```python
from build123d import *

# Parameters (mm, degrees)
SKETCH1_R             = 1.6499999999999988
SKETCH1_R_2           = 1.6499999999999992
BOSS_EXTRUDE1_DEPTH   = 24
BOSS_EXTRUDE1_2_DEPTH = 24
SKETCH5_R             = 3.0000000000000044
SKETCH5_R_2           = 2.9999999999999996
CUT_EXTRUDE1_DEPTH    = 3
SKETCH6_W             = 2.999999999999975
SKETCH6_H             = 17.999999999999996
BOSS_EXTRUDE2_DEPTH   = 5
FILLET1_R             = 3
BOSS_EXTRUDE3_DEPTH   = 7
CHAMFER1_SIZE         = 2
FILLET2_R             = 0.6
FILLET3_R             = 1.2
CHAMFER2_SIZE         = 0.2
FILLET4_R             = 0.8


with BuildPart() as part:
    # Sketch1 → Boss-Extrude1 (new body)
    with BuildSketch(Plane.XY):
        with BuildLine():
            Line((-24.12157620169872, 10.3), (-9.293008124391159, 10.3))
            ThreePointArc((-9.293008124391159, 10.3), (-9.052493629563461, 10.342616719274229), (-8.841264673899918, 10.465277777777773))
            ThreePointArc((-8.84126467389991, 10.465277777777777), (-2.7566148708280886, 13.419801580274177), (4.000000000000017, 13.103053079339933))
            Line((4.000000000000019, 13.103053079339944), (4.000000000000019, 18))
            ThreePointArc((4.0000000000000195, 18), (1.4019415263376545, 21.7462728086366), (-3.0172799783650257, 20.626027709708623))
            ThreePointArc((-3.017279978365025, 20.626027709708623), (-5.396557983146459, 18.850985983990057), (-8.297519940503818, 18.221576201698717))
            Line((-8.297519940503818, 18.22157620169872), (-22, 18.221576201698717))
            ThreePointArc((-22, 18.221576201698717), (-26.540740078127286, 16.340740078127293), (-28.42157620169869, 11.799999999999997))
            Line((-28.42157620169869, 11.799999999999997), (-28.421576201698695, 8.999999999999998))
            Line((-28.421576201698695, 8.999999999999998), (-25.42157620169872, 8.999999999999998))
            ThreePointArc((-25.42157620169872, 8.999999999999998), (-25.040815017241233, 9.919238815542512), (-24.12157620169872, 10.3))
        make_face()
        with Locations((-21.999999999999996, 14)):
            Circle(SKETCH1_R, mode=Mode.SUBTRACT)
        with Locations((-6.49e-15, 18)):
            Circle(SKETCH1_R_2, mode=Mode.SUBTRACT)
    extrude(amount=BOSS_EXTRUDE1_DEPTH)


with BuildPart() as body_2:
    # Sketch1 → Boss-Extrude1 2 (new body)
    with BuildSketch(Plane.XY):
        with BuildLine():
            ThreePointArc((-24.12157620169872, -10.299999999999999), (-25.040815017241233, -9.91923881554251), (-25.42157620169872, -8.999999999999998))
            Line((-25.42157620169872, -8.999999999999998), (-28.421576201698723, -8.999999999999998))
            Line((-28.421576201698723, -8.999999999999998), (-28.42157620169872, -11.799999999999997))
            ThreePointArc((-28.42157620169872, -11.799999999999997), (-26.540740078127314, -16.340740078127318), (-21.999999999999996, -18.22157620169873))
            Line((-21.999999999999996, -18.22157620169873), (-8.297519940503813, -18.221576201698728))
            ThreePointArc((-8.297519940503813, -18.221576201698728), (-5.3965579831464545, -18.850985983990064), (-3.0172799783650195, -20.62602770970863))
            ThreePointArc((-3.0172799783650204, -20.62602770970863), (1.4019415263376571, -21.74627280863661), (4.000000000000004, -18))
            Line((4.000000000000004, -18), (4.000000000000004, -13.103053079339944))
            ThreePointArc((4.000000000000004, -13.103053079339945), (-2.756614870828109, -13.41980158027418), (-8.841264673899921, -10.465277777777775))
            ThreePointArc((-8.841264673899923, -10.465277777777775), (-9.052493629563463, -10.342616719274227), (-9.293008124391159, -10.299999999999999))
            Line((-9.293008124391159, -10.299999999999999), (-24.12157620169872, -10.299999999999999))
        make_face()
        with Locations((-21.999999999999996, -14)):
            Circle(SKETCH1_R, mode=Mode.SUBTRACT)
        with Locations((4.53e-15, -18)):
            Circle(SKETCH1_R_2, mode=Mode.SUBTRACT)
    extrude(amount=BOSS_EXTRUDE1_2_DEPTH)


with BuildPart() as cut_extrude1_tool:
    # Sketch5 → Cut-Extrude1 (new body)
    with BuildSketch(Plane.XY.offset(24)):
        with Locations((-21.999999999999996, 14)):
            Circle(SKETCH5_R)
        with Locations((-6.49e-15, 18)):
            Circle(SKETCH5_R_2)
        with Locations((4.53e-15, -18)):
            Circle(SKETCH5_R_2)
        with Locations((-21.999999999999996, -14)):
            Circle(SKETCH5_R)
    extrude(amount=-CUT_EXTRUDE1_DEPTH)


with BuildPart() as part_1:
    add(part.part)

    # Cut-Extrude1: cut by cut_extrude1_tool
    add(cut_extrude1_tool.part, mode=Mode.SUBTRACT)



with BuildPart() as body_2_1:
    add(body_2.part)

    # Cut-Extrude1: cut by cut_extrude1_tool
    add(cut_extrude1_tool.part, mode=Mode.SUBTRACT)


with BuildPart() as part_2:
    add(part_1.part)

    add(body_2_1.part)  # Boss-Extrude2 merges body 2
    # Sketch6 → Boss-Extrude2 (add)
    with BuildSketch(Plane.XY.offset(24)):
        with Locations((-26.921576201698706, 0)):
            Rectangle(SKETCH6_W, SKETCH6_H)
    extrude(amount=-BOSS_EXTRUDE2_DEPTH)

    # Fillet1
    fillet1_edges = [part_2.edges().sort_by_distance(p)[0] for p in [
        (4.000000000000018, 13.103053079339938, 12),
        (4.0000000000000036, -13.103053079339944, 12),
    ]]
    fillet(fillet1_edges, radius=FILLET1_R)

    # Sketch7 → Boss-Extrude3 (add)
    with BuildSketch(Plane.XY.offset(24)):
        Polygon((-28.42157620169872, 8.000000000000004), (-25.42157620169872, 8.000000000000004), (-25.42157620169872, -7.9999999999999964), (-28.421576201698716, -7.9999999999999964), align=None)
        with BuildLine():
            Line((-17.999999999999996, 10.3), (-9.293008124391159, 10.3))
            ThreePointArc((-9.293008124391159, 10.3), (-9.052493629563465, 10.342616719274229), (-8.841264673899923, 10.465277777777771))
            ThreePointArc((-8.841264673899923, 10.465277777777771), (-6.554691773201115, 12.030212623155485), (-4, 13.103053079339944))
            Line((-4, 13.103053079339944), (-3.999999999999999, 16.21388294024599))
            ThreePointArc((-3.999999999999999, 16.21388294024599), (-7.198728243522483, 15.068786005379188), (-10.099504938362077, 13.299999999999999))
            Line((-10.099504938362077, 13.299999999999999), (-17.999999999999996, 13.299999999999999))
            Line((-17.999999999999996, 13.299999999999999), (-17.999999999999996, 10.3))
        make_face()
        with BuildLine():
            Line((-17.999999999999993, -10.300000000000004), (-9.293008124391159, -10.3))
            ThreePointArc((-9.293008124391159, -10.3), (-9.052493629563465, -10.342616719274229), (-8.841264673899923, -10.465277777777771))
            ThreePointArc((-8.841264673899923, -10.465277777777771), (-6.554691773201115, -12.030212623155485), (-4, -13.103053079339944))
            Line((-4, -13.103053079339944), (-3.9999999999999947, -16.21388294024599))
            ThreePointArc((-3.9999999999999947, -16.21388294024599), (-7.198728243522483, -15.068786005379188), (-10.099504938362074, -13.300000000000002))
            Line((-10.099504938362074, -13.300000000000002), (-17.999999999999993, -13.300000000000002))
            Line((-17.999999999999993, -13.300000000000002), (-17.999999999999993, -10.300000000000004))
        make_face()
    extrude(amount=BOSS_EXTRUDE3_DEPTH)

    # Chamfer1
    chamfer1_edges = [part_2.edges().sort_by_distance(p)[0] for p in [
        (-28.42157620169872, 3.55e-15, 31),
    ]]
    chamfer(chamfer1_edges, length=CHAMFER1_SIZE)

    # Fillet2
    fillet2_edges = [part_2.edges().sort_by_distance(p)[0] for p in [
        (-25.42157620169872, -7.9999999999999964, 27.5),
        (-25.42157620169872, 8.000000000000004, 27.5),
        (-17.999999999999996, 13.299999999999999, 27.5),
        (-17.999999999999996, 10.3, 27.5),
        (-3.9999999999999996, 13.103053079339945, 27.5),
        (-10.099504938362077, 13.299999999999999, 27.5),
        (-17.999999999999993, -10.300000000000004, 27.5),
        (-17.999999999999993, -13.300000000000002, 27.5),
        (-10.099504938362076, -13.3, 27.5),
        (-3.9999999999999996, -13.103053079339945, 27.5),
        (-28.421576201698716, -7.9999999999999964, 26.5),
        (-28.42157620169872, 8.000000000000004, 26.499999999999993),
    ]]
    fillet(fillet2_edges, radius=FILLET2_R)

    # Fillet3
    fillet3_edges = [part_2.edges().sort_by_distance(p)[0] for p in [
        (-3.999999999999999, 16.213882940245995, 27.5),
        (-3.9999999999999947, -16.21388294024599, 27.5),
    ]]
    fillet(fillet3_edges, radius=FILLET3_R)

    # Chamfer2
    chamfer2_edges = [part_2.edges().sort_by_distance(p)[0] for p in [
        (-23.649999999999995, 14, 21),
        (-1.6500000000000057, 18, 21),
        (-23.649999999999995, -14, 21),
        (-1.6499999999999948, -18, 21),
    ]]
    chamfer(chamfer2_edges, length=CHAMFER2_SIZE)

    # Fillet4
    fillet4_edges = [part_2.edges().sort_by_distance(p)[0] for p in [
        (-25.42157620169872, 8.999999999999998, 9.5),
        (-28.421576201698695, 8.999999999999998, 9.5),
        (-25.42157620169872, -8.999999999999998, 9.5),
        (-28.421576201698723, -8.999999999999998, 9.5),
    ]]
    fillet(fillet4_edges, radius=FILLET4_R)


solid = part_2.part
```
For this review, take the finished solid that the model builds, in its own axes (mm). A direction names the side the tool comes from. Coordinates: 2 decimals unless noted, no trailing zeros. Loops run counter-clockwise (first coordinate to the right, second up) from the corner with the lowest first, then second, coordinate; pieces in that order, holes last. Notation, with made-up numbers: (-2, -33) -> (41, -33) arc R25 cw to (41, -3) -> close; hole circle Ø7 at (19.5, 33). An arc over 180 degrees is marked (long way). Return JSON: item names as keys, results as strings. Group by question number.
(1) Tool access review of faces 4 (the cylindrical face through (1.47, 21.72, 11.83)), 5 (the cylindrical face through (-4.52, -15.59, 27.55)), 6 (the cylindrical face through (-0.65, -20.93, 22.52)), 7 (the cylindrical face through (-4.52, 15.59, 27.55)), 8 (the cylindrical face through (-24.879, 10.057, 11.832)): name each direction out of +Z, -Z, +X, -X, +Y, -Y from which nothing blocks a thin tool from reaching the whole face with its end or side.
(2) Consider section B-B, the plane x = 0. Give the boundary of the cut face in (y, z).
(3) For pin 1 Ø2 at (x, z) = (-15.5, 28.5) entering from +Y; pin 2 Ø6.5 at (x, y) = (-22.5, -13) entering from +Z; pin 3 Ø4.5 at (x, y) = (0, 18) entering from +Z; pin 4 Ø11.5 at (x, y) = (-6, -16.5) entering from +Z, all flat-tipped, find the tip position at first contact; note any pin that passes through.
(4) Mouldability with a two-part tool opening along Y and no side actions: class faces 1 (the cylindrical face through (-26.49, 16.39, 11.83)), 2 (the flat face through (-22, 12, 21)), 3 (the flat face through (-14, -13.3, 27)) as pulls with the +Y half, pulls with the -Y half, needs draft (parallel to the pull), parting line crosses it, or undercut.
(5) To check wall thickness, follow L1, parallel to Y at x = 0, z = 6; L2, parallel to Y at x = -15.5, z = 25; L3, parallel to Y at x = -17.5, z = 17. State the ranges of each line that lie inside material, in increasing order.
(6) Consider section A-A, the plane z = 26. Count the separate pieces of the cut face and the enclosed holes in it, plus the area to 3 significant figures.
(7) Consider section D-D, the plane y = -2. Give the boundary of the cut face in (x, z).
Results below:
{
 "1": {"face 4": "+Z, -Z, +Y", "face 5": "+Z, -Y", "face 6": "+Z", "face 7": "+Z, +Y", "face 8": "+Z, -Z, +X"},
 "2": {"outline": "(-22, 0) -> (-19.65, 0) -> (-19.65, 20.8) -> (-19.85, 21) -> (-21, 21) -> (-21, 24) -> (-22, 24) -> close; (-16.35, 0) -> (-13.7, 0) -> (-13.7, 24) -> (-15, 24) -> (-15, 21) -> (-16.15, 21) -> (-16.35, 20.8) -> close; (13.7, 0) -> (16.35, 0) -> (16.35, 20.8) -> (16.15, 21) -> (15, 21) -> (15, 24) -> (13.7, 24) -> close; (19.65, 0) -> (22, 0) -> (22, 24) -> (21, 24) -> (21, 21) -> (19.85, 21) -> (19.65, 20.8) -> close"},
 "3": {"pin 1": "stops at y = 13.3", "pin 2": "stops at z = 24", "pin 3": "stops at z = 21", "pin 4": "stops at z = 31"},
 "4": {"face 1": "pulls with the +Y half", "face 2": "undercut", "face 3": "pulls with the -Y half"},
 "5": {"L1": "y = -22 to -19.65, -16.35 to -13.7, 13.7 to 16.35, 19.65 to 22", "L2": "y = -13.3 to -10.3, 10.3 to 13.3", "L3": "y = -18.22 to -10.3, 10.3 to 18.22"},
 "6": {"separate pieces": "3", "enclosed holes": "0", "area": "135 mm2"},
 "7": {"outline": "(-28.42, 19) -> (-25.42, 19) -> (-25.42, 31) -> (-26.42, 31) -> (-28.42, 29) -> close"}
}
